Autodesk Inventor part; units mm, degrees
ref_plane "YZ Plane" through (0, 0, 0) normal (1, 0, 0) x (0, 1, 0)
ref_plane "XZ Plane" through (0, 0, 0) normal (0, 1, 0) x (-1, 0, 0)
ref_plane "XY Plane" through (0, 0, 0) normal (0, 0, 1) x (1, 0, 0)
sketch "Sketch1" plane through (0, 0, 0) normal (0, 0, 1) x (1, 0, 0)
  line L0 (0, 0) -> (-50.8, 0)
  line L1 (-50.8, 0) -> (-50.8, -101.6)
  line L2 (-50.8, -101.6) -> (0, -101.6)
  line L3 (0, -22.225) -> (-38.1, -22.225)
  line L4 (-38.1, -22.225) -> (-38.1, -41.275)
  line L5 (-38.1, -41.275) -> (0, -41.275)
  line L6 (0, -101.6) -> (0, -41.275)
  line L7 (0, -22.225) -> (0, 0)
  dimension "d0" = 101.6
  dimension "d1" = 50.8
  dimension "d4" = 22.225
  dimension "d5" = 38.1
  dimension "d6" = 19.05
extrude "Extrusion1" add sketch "Sketch1" along normal blind 44.45
sketch "Sketch2" plane through (0, -22.225, 0) normal (1, 0, 0) x (0, 0, -1)
  line L0 (-44.45, 0) -> (-44.45, 22.225)
  line L1 (0, 22.225) -> (0, -79.375)
  line L2 (-44.45, 22.225) -> (0, 22.225)
  line L3 (0, 22.225) -> (0, -79.375)
  line L4 (0, -79.375) -> (-44.45, -79.375)
  line L5 (-44.45, -79.375) -> (-44.45, 22.225)
extrude "Extrusion2" cut sketch "Sketch2" against normal blind 0.381
sketch "Sketch3" plane through (-50.8, 0, 44.45) normal (0, 1, 0) x (1, 0, 0)
  line L0 (0, 44.45) -> (0, 0)
  line L1 (50.419, 44.45) -> (0, 44.45)
  point P0 (50.8, 44.45)
  point P1 (38.1, 22.225)
  dimension "d9" = 38.1
  dimension "d10" = 22.225
hole "Hole1" at (-12.7, 0, 22.225) direction (0, -1, 0) diameter 6.7564 end up to surface
sketch "Sketch4" plane through (-50.8, -101.6, 0) normal (-1, 0, 0) x (0, 0, 1)
  line L0 (0, 101.6) -> (0, 0)
  line L1 (0, 101.6) -> (44.45, 101.6)
  point P0 (22.225, 69.85)
  dimension "d18" = 22.225
  dimension "d19" = 31.75
hole "Hole2" at (-50.8, -31.75, 22.225) direction (1, 0, 0) diameter 6.7564 end through all
sketch "Sketch5" plane through (-50.8, -101.6, 0) normal (-1, 0, 0) x (0, 0, 1)
  line L0 (0, 101.6) -> (0, 0)
  line L1 (0, 101.6) -> (44.45, 101.6)
  point P0 (15.875, 31.75)
  dimension "d27" = 15.875
  dimension "d28" = 69.85
hole "Hole3" at (-50.8, -69.85, 15.875) direction (1, 0, 0) diameter 25.4 end through all
sketch "Sketch6" plane through (0, 0, 44.45) normal (0, 0, 1) x (1, 0, 0)
  line L0 (-0.381, 0) -> (-50.8, 0)
  line L1 (-50.8, 0) -> (-50.8, -101.6)
  point P0 (0, 0)
  point P1 (-25.4, -69.85)
  dimension "d36" = 69.85
  dimension "d37" = 25.4
hole "Hole4" at (-25.4, -69.85, 44.45) direction (0, 0, -1) diameter 6.7564 end through all
sketch "Sketch7" plane through (0, 0, 44.45) normal (0, 0, 1) x (1, 0, 0)
  circle A0 centre (-25.4, -107.95) radius 20.32
  line L0 (-0.381, 0) -> (-50.8, 0)
  line L1 (-50.8, 0) -> (-50.8, -101.6)
  point P0 (0, 0)
  dimension "d45" = 107.95
  dimension "d46" = 25.4
  dimension "d47" = 40.64
extrude "Extrusion3" cut sketch "Sketch7" against normal through all
properties part number "RM Over Support For Arm With Delrin Slider"
Geometry: final body of the model. Coordinates: model frame, mm. A direction names the side the tool comes from. Coordinates: 2 decimals unless noted, no trailing zeros. Order: outer loops, then holes, each group sorted by start corner. A loop starts at its lowest first (then second) coordinate and runs counter-clockwise, first axis right, second up.
(1) Section query A-A (y = -31.75). Return the cut outline in (x, z).
(2) Draft query along X for faces 1 (the face through (-19, -22.225, 22)), 2 (the face through (-25.549, -66.475, 1.791)), 3 (the face through (-38.1, -36, 22)). Return one class per face: pulls with the +X half, pulls with the -X half, needs draft (parallel to the pull), parting line crosses it, or undercut.
(3) Section query D-D (x = -32). Return the cut outline in (y, z) (3 decimals), plus the area to 3 significant figures.
(4) Access query for faces 4 (the face through (-20, -41.275, 22)), 5 (the face through (-25.24, -73.66, 27.99)), 6 (the face through (-10.644, -11.268, 19.544)). Directions: +Z, -Z, +X, -X, +Y, -Y. A direction counts if a zero-diameter tool reaches every point of the face in a straight line with its end or side. Return the directions, or none.
(5) Material intervals for probe 1 along Y at (x, z) = (-2.5, 14.5) (3 decimals); probe 2 along Z at (x, y) = (-41, -31.75); probe 3 along Y at (x, z) = (-28, 24) (3 decimals), sorted ascending.
(6) First-contact query: pin 1 (5.5 mm diameter, centred on y = -28.5, z = 26.5, fed in from +X); pin 2 (19 mm diameter, centred on x = -18, z = 26.5, fed in from -Y); pin 3 (9 mm diameter, centred on x = -12.7, z = 22.225, fed in from -Y). Flat tips, straight axial feed; report the tip coordinate or a pass-through.
(7) Section query B-B (x = -12.7). Return the cut outline in (y, z) (3 decimals).
(8) Section query C-C (y = -69.85). Return the cut outline in (x, z) (3 decimals).
Solution:
1. outline: (-50.8, 0) - (-38.1, 0) - (-38.1, 18.85) - (-50.8, 18.85) - close; (-50.8, 25.6) - (-38.1, 25.6) - (-38.1, 44.45) - (-50.8, 44.45) - close
2. face 1: needs draft
2. face 2: undercut
2. face 3: pulls with the +X half
3. outline: (-88.732, 0) - (-41.275, 0) - (-41.275, 44.45) - (-88.732, 44.45) - close; (-22.225, 0) - (0, 0) - (0, 44.45) - (-22.225, 44.45) - close; hole circle Ø25.4 at (-69.85, 15.875)
3. area: 2,590 mm2
4. face 4: +Z, -Z, +X
4. face 5: +X, -X
4. face 6: +Y
5. probe 1: y = -101.6 to -82.475, -57.225 to -41.275, -22.225 to 0
5. probe 2: z = 0 to 18.85, 25.6 to 44.45
5. probe 3: y = -87.797 to -79.611, -60.089 to -41.275, -22.225 to 0
6. pin 1: stops at x = -38.1
6. pin 2: stops at y = -96.67
6. pin 3: stops at y = -97.13
7. outline: (-92.088, 0) - (-41.275, 0) - (-41.275, 44.45) - (-92.088, 44.45) - close; (-22.225, 0) - (0, 0) - (0, 18.847) - (-22.225, 18.847) - close; (-22.225, 25.603) - (0, 25.603) - (0, 44.45) - (-22.225, 44.45) - close; hole circle Ø25.4 at (-69.85, 15.875)
8. outline: (-50.8, 0) - (-28.778, 0) - (-28.778, 3.175) - (-50.8, 3.175) - close; (-50.8, 28.575) - (-28.778, 28.575) - (-28.778, 44.45) - (-50.8, 44.45) - close; (-22.022, 0) - (-0.381, 0) - (-0.381, 3.175) - (-22.022, 3.175) - close; (-22.022, 28.575) - (-0.381, 28.575) - (-0.381, 44.45) - (-22.022, 44.45) - close
